from build123d import *

# Parameters (mm, degrees)
SKETCH_1_R      = 2.5
EXTRUDE_1_DEPTH = 5


with BuildPart() as part:
    # 草图1 → 凸台-拉伸1 (new body)
    with BuildSketch(Plane.XY.offset(5)):
        with BuildLine():
            Line((12, -47.16), (12, 47.16))
            ThreePointArc((12, 47.16), (0, 59.16), (-12, 47.16))
            Line((-12, 47.16), (-12, -47.16))
            ThreePointArc((-12, -47.16), (0, -59.16), (12, -47.16))
        make_face()
        with Locations(Location((0, -47.16, 0), (0, 0, 180))):
            Circle(SKETCH_1_R, mode=Mode.SUBTRACT)
        with Locations(Location((0, 47.16, 0), (0, 0, 180))):
            Circle(SKETCH_1_R, mode=Mode.SUBTRACT)
    extrude(amount=-EXTRUDE_1_DEPTH)


solid = part.part
Could you check a few things on this model? Use its own coordinates, in mm. Give positions to 0.01 mm unless a question says otherwise; leave off trailing zeros. Order: outer loops, then holes, each group sorted by start corner. A loop starts at its lowest first (then second) coordinate and runs counter-clockwise, first axis right, second up. Notation, with made-up numbers: (-7, -36.75) - (42, -36.75) arc R22 ccw to (42, -27.75) - close; hole circle Ø11 at (84, -3.5). An arc over 180 degrees is marked (long way). One line per item, written item: value. Start each with the question number.
1. Imagine slicing it at C-C on x = -8.5. List the corners of the cut face in (y, z) for me, plus the area to 3 significant figures.
2. Imagine slicing it at B-B on z = 3. List the corners of the cut face in (x, y) for me.
3. Imagine slicing it at D-D on x = 5. List the corners of the cut face in (y, z) for me, plus the area to 3 significant figures.
4. Thinking about a two-plate mould opening in Y: for faces 1 (the face through (0.54, -44.72, 2.54)), 2 (the face through (-0.264, -59.157, 2.535)), 3 (the face through (0, 1, 0)), 4 (the face through (0.33, 44.68, 2.54)), which applies, +Y half, -Y half, draft (parallel to the pull), parting line (faces both ways), or undercut?
5. Imagine slicing it at A-A on x = 0. List the corners of the cut face in (y, z) for me.
6. If I drill on probe 1 along Y at (x, z) = (0, 3); probe 2 along Y at (x, z) = (0.25, 2.95); probe 3 along X at (y, z) = (-47.16, 3.3), over which ranges is the centre line in solid material (lowest first)?
Values:
1. outline: (-55.63, 0) - (55.63, 0) - (55.63, 5) - (-55.63, 5) - close
1. area: 556 mm²
2. outline: (-12, -47.16) arc R12 ccw to (12, -47.16) - (12, 47.16) arc R12 ccw to (-12, 47.16) - close; hole circle Ø5 at (0, -47.16); hole circle Ø5 at (0, 47.16)
3. outline: (-58.07, 0) - (58.07, 0) - (58.07, 5) - (-58.07, 5) - close
3. area: 581 mm²
4. face 1: undercut
4. face 2: -Y half
4. face 3: draft
4. face 4: undercut
5. outline: (-59.16, 0) - (-49.66, 0) - (-49.66, 5) - (-59.16, 5) - close; (-44.66, 0) - (44.66, 0) - (44.66, 5) - (-44.66, 5) - close; (49.66, 0) - (59.16, 0) - (59.16, 5) - (49.66, 5) - close
6. probe 1: -59.16 to -49.66, -44.66 to 44.66, 49.66 to 59.16
6. probe 2: -59.16 to -49.65, -44.67 to 44.67, 49.65 to 59.16
6. probe 3: -12 to -2.5, 2.5 to 12
